Verification items for the finished model (mm, model axes). A direction names the side the tool comes from. Coordinates: 2 decimals unless noted, no trailing zeros.
Q1. Cross-section at A-A, the plane z = 11.5. Count the separate pieces of the cut face and the enclosed holes in it, and give its area (3 significant figures).
Q2. Set-up check for faces 5 (the cylindrical face through (-30.235, -23.183, 12.789)), 6 (the flat face through (27.3, -27.3, 19.05)): record each of +Z, -Z, +X, -X, +Y, -Y from which the full face is reachable in a straight line by a thin tool's end or side.
Q3. Thickness scan on line 1 (Y direction, x = 0, z = 11) (3 decimals); line 2 (Y direction, x = -4.5, z = 17.5); line 3 (X direction, y = -42.5, z = 13.25). Record the ranges inside material, lowest first.
Q4. Draft check along Y on faces 1 (the cylindrical face through (21.199, 6.676, 12.789)), 2 (the flat face through (-1, 1, 0)), 3 (the cylindrical face through (-13.77, -61.99, 9.39)), 4 (the flat face through (16, -16, 6.35)). Enter one of: pulls with the +Y half, pulls with the -Y half, needs draft (parallel to the pull), parting line crosses it, or undercut.
Q5. Depth check by flat-ended pin: P1, Ø6, axis at y = 43.5, z = 11.5, coming from the +X side; P2, Ø1, axis at x = -2, z = 6.5, coming from the +Y side; P3, Ø3, axis at x = 34, y = -3, coming from the +Z side. Enter the tip coordinate at first touch or a pass-through.
from build123d import *

# Parameters (mm, degrees)
F0_R     = 63.5
F1_DEPTH = 19.05
F2_R     = 38.1
F2_R_2   = 22.225
F3_DEPTH = 12.7
F5_DEPTH = 25.4
F7_DEPTH = 25.4


with BuildPart() as f1:
    # F0 (on Top) → F1 (new body)
    with BuildSketch(Plane.XY):
        Circle(F0_R)
    extrude(amount=F1_DEPTH)

    # F2 (on face) → F3 (cut)
    with BuildSketch(Plane.XY.offset(19.05)):
        Circle(F2_R)
        Circle(F2_R_2, mode=Mode.SUBTRACT)
    extrude(amount=-F3_DEPTH, mode=Mode.SUBTRACT)

    # F4 (on face) → F5 (cut)
    with BuildSketch(Plane.XY.offset(19.05)):
        with BuildLine():
            ThreePointArc((-53.975, 0), (-54.873968, 2.213663), (-57.061806, 3.173775))
            ThreePointArc((-57.061806, 3.173775), (-60.325, 0), (-57.061806, -3.173775))
            ThreePointArc((-57.061806, -3.173775), (-54.873968, -2.213663), (-53.975, 0))
        make_face()
        with BuildLine():
            ThreePointArc((-38.104592, 42.592987), (-42.656217, 42.656217), (-42.592987, 38.104592))
            ThreePointArc((-42.592987, 38.104592), (-39.155505, 37.494995), (-37.236153, 40.411153))
            ThreePointArc((-37.236153, 40.411153), (-37.461241, 41.585311), (-38.104592, 42.592987))
        make_face()
        with BuildLine():
            ThreePointArc((3.175, 57.15), (-0.044101, 60.324694), (-3.173775, 57.061806))
            ThreePointArc((-3.173775, 57.061806), (0, 53.975), (3.173775, 57.061806))
            ThreePointArc((3.173775, 57.061806), (3.174694, 57.105899), (3.175, 57.15))
        make_face()
        with BuildLine():
            ThreePointArc((43.586153, 40.411153), (41.585311, 43.361064), (38.104592, 42.592987))
            ThreePointArc((38.104592, 42.592987), (38.166089, 38.166089), (42.592987, 38.104592))
            ThreePointArc((42.592987, 38.104592), (43.32731, 39.155505), (43.586153, 40.411153))
        make_face()
        with BuildLine():
            ThreePointArc((60.325, 0), (59.363663, 2.276032), (57.061806, 3.173775))
            ThreePointArc((57.061806, 3.173775), (53.975, 0), (57.061806, -3.173775))
            ThreePointArc((57.061806, -3.173775), (59.363663, -2.276032), (60.325, 0))
        make_face()
        with BuildLine():
            ThreePointArc((42.592987, -38.104592), (38.166089, -38.166089), (38.104592, -42.592987))
            ThreePointArc((38.104592, -42.592987), (41.585311, -43.361064), (43.586153, -40.411153))
            ThreePointArc((43.586153, -40.411153), (43.32731, -39.155505), (42.592987, -38.104592))
        make_face()
        with BuildLine():
            ThreePointArc((3.173775, -57.061806), (0, -53.975), (-3.173775, -57.061806))
            ThreePointArc((-3.173775, -57.061806), (-0.044101, -60.324694), (3.175, -57.15))
            ThreePointArc((3.175, -57.15), (3.174694, -57.105899), (3.173775, -57.061806))
        make_face()
        with BuildLine():
            ThreePointArc((-37.236153, -40.411153), (-39.155505, -37.494995), (-42.592987, -38.104592))
            ThreePointArc((-42.592987, -38.104592), (-42.656217, -42.656217), (-38.104592, -42.592987))
            ThreePointArc((-38.104592, -42.592987), (-37.461241, -41.585311), (-37.236153, -40.411153))
        make_face()
    extrude(amount=-F5_DEPTH, mode=Mode.SUBTRACT)

    # F6 (on face) → F7 (cut)
    with BuildSketch(Plane.XY.offset(6.35)):
        with BuildLine():
            ThreePointArc((-29.36875, 0), (-29.597554, 0.557561), (-30.152056, 0.793681))
            ThreePointArc((-30.152056, 0.793681), (-30.95625, 0), (-30.152056, -0.793681))
            ThreePointArc((-30.152056, -0.793681), (-29.597554, -0.557561), (-29.36875, 0))
        make_face()
        with BuildLine():
            ThreePointArc((0.793681, -30.152056), (0, -29.36875), (-0.793681, -30.152056))
            ThreePointArc((-0.793681, -30.152056), (-0.005222, -30.956233), (0.79375, -30.1625))
            ThreePointArc((0.79375, -30.1625), (0.793733, -30.157278), (0.793681, -30.152056))
        make_face()
        with BuildLine():
            ThreePointArc((30.95625, 0), (30.720061, 0.564946), (30.152056, 0.793681))
            ThreePointArc((30.152056, 0.793681), (29.36875, 0), (30.152056, -0.793681))
            ThreePointArc((30.152056, -0.793681), (30.720061, -0.564946), (30.95625, 0))
        make_face()
        with BuildLine():
            ThreePointArc((0.79375, 30.1625), (-0.005222, 30.956233), (-0.793681, 30.152056))
            ThreePointArc((-0.793681, 30.152056), (0, 29.36875), (0.793681, 30.152056))
            ThreePointArc((0.793681, 30.152056), (0.793733, 30.157278), (0.79375, 30.1625))
        make_face()
    extrude(amount=-F7_DEPTH, mode=Mode.SUBTRACT)


solid = f1.part
Check values:
1. separate pieces: 2
1. enclosed holes: 9
1. area: 9,410 mm2
2. face 5: +Z
2. face 6: +Z, +X, -X, +Y, -Y
3. line 1: y = -63.5 to -60.325, -53.975 to -38.1, -22.225 to 22.225, 38.1 to 53.975, 60.325 to 63.5
3. line 2: y = -63.34 to -37.83, -21.76 to 21.76, 37.83 to 63.34
3. line 3: x = -47.18 to -42.8, -38.02 to 38.02, 42.8 to 47.18
4. face 1: undercut
4. face 2: needs draft
4. face 3: parting line crosses it
4. face 4: undercut
5. P1: stops at x = 48.91
5. P2: stops at y = 63.48
5. P3: stops at z = 6.35
